Could you check a few things on this model? Use its own coordinates, in mm. Face numbers are marked on the shaded views. A direction names the side the tool comes from. Coordinates: 2 decimals unless noted, no trailing zeros. Loops run counter-clockwise (first coordinate to the right, second up) from the corner with the lowest first, then second, coordinate; pieces in that order, holes last. Notation, with made-up numbers: (59, 60) - (117, 60) arc R25 ccw to (117, 75) - close; hole circle Ø2 at (41.25, 7.5). An arc over 180 degrees is marked (long way). Use CSV: the item, a comma, the result in double quotes.
from build123d import *

# Parameters (mm, degrees)
CROQUIS1_R              = 13.75
SALIENTE_EXTRUIR1_DEPTH = 27
CROQUIS3_R              = 1.6
SALIENTE_EXTRUIR2_DEPTH = 11.5
REDONDEO1_R             = 2


with BuildPart() as part:
    # Croquis1 → Saliente-Extruir1 (new body)
    with BuildSketch(Plane(origin=(0, 0, 0), x_dir=(1, 0, 0), z_dir=(0, 1, 0))):
        with Locations(Location((0, 0, 0), (0, 0, 270))):
            Circle(CROQUIS1_R)
    extrude(amount=SALIENTE_EXTRUIR1_DEPTH)

    # Croquis3 → Saliente-Extruir2 (add)
    with BuildSketch(Plane(origin=(0, 27, 0), x_dir=(1, 0, 0), z_dir=(0, 1, 0))):
        with Locations(Location((0, 0, 0), (0, 0, 270))):
            Circle(CROQUIS3_R)
    extrude(amount=SALIENTE_EXTRUIR2_DEPTH)

    # Redondeo1
    redondeo1_edges = [part.edges().sort_by_distance(p)[0] for p in [
        (0, 0, -13.75),
        (0, 27, -13.75),
        (0, 27, -1.6),
    ]]
    fillet(redondeo1_edges, radius=REDONDEO1_R)


solid = part.part
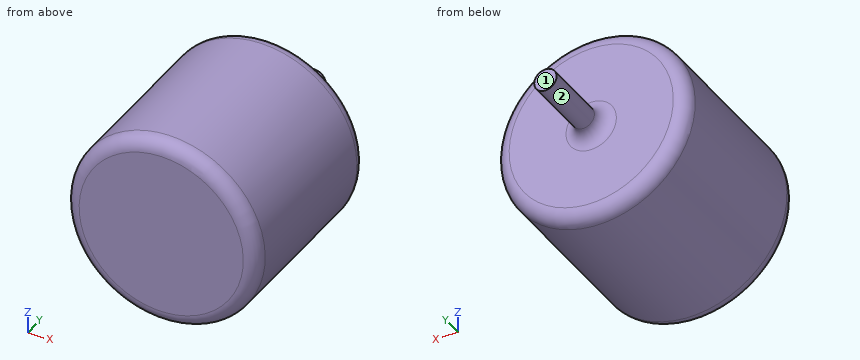
(1) Suppose I cut it at C-C (y = 11.5). Write out the boundary of the cut face in (x, z), plus the area to 3 significant figures.
Computed:
outline,"circle Ø27.5 at (0, 0)"
area,"594 mm²"
(2) Please list where these lines run through material, in increasing order: line 1 (Y direction, x = 2, z = -9.5); line 2 (Z direction, x = -0.5, y = 14.5); line 3 (X direction, y = 14.5, z = 9.5).
Computed:
line 1,"y = 0 to 27"
line 2,"z = -13.74 to 13.74"
line 3,"x = -9.94 to 9.94"
(3) Suppose I cut it at B-B (z = 0). Write out the boundary of the cut face in (x, y).
Computed:
outline,"(-13.75, 2) arc R2 ccw to (-11.75, 0) - (11.75, 0) arc R2 ccw to (13.75, 2) - (13.75, 25) arc R2 ccw to (11.75, 27) - (3.6, 27) arc R2 cw to (1.6, 29) - (1.6, 38.5) - (-1.6, 38.5) - (-1.6, 29) arc R2 cw to (-3.6, 27) - (-11.75, 27) arc R2 ccw to (-13.75, 25) - close"
(4) Will these pins go through, and if not, where does the flat tip stop? pin 1 (2 mm diameter, centred on x = -5, y = 16, fed in from -Z); pin 2 (4 mm diameter, centred on x = 10.5, y = 19.5, fed in from -Z); pin 3 (2 mm diameter, centred on y = 24.5, z = -9.5, fed in from +X).
Computed:
pin 1,"stops at z = -13.16"
pin 2,"stops at z = -10.81"
pin 3,"stops at x = 10.81"
(5) Suppose I cut it at A-A (x = 0). Write out the boundary of the cut face in (y, z), plus the area to 3 significant figures.
Computed:
outline,"(0, -11.75) arc R2 ccw to (2, -13.75) - (25, -13.75) arc R2 ccw to (27, -11.75) - (27, -3.6) arc R2 cw to (29, -1.6) - (38.5, -1.6) - (38.5, 1.6) - (29, 1.6) arc R2 cw to (27, 3.6) - (27, 11.75) arc R2 ccw to (25, 13.75) - (2, 13.75) arc R2 ccw to (0, 11.75) - close"
area,"778 mm²"
(6) Which directions (+Z, -Z, +X, -X, +Y, -Y) give clear straight access to the entire face, cutting with the end or side of a thin tool? Please do the marked faces 1 and 2.
Computed:
face 1,"+Z, -Z, +X, -X, +Y"
face 2,"+Y"
